from build123d import *

# Parameters (mm, degrees)
SKETCH1_W           = 100
SKETCH1_H           = 320
SKETCH1_R           = 1.6
SKETCH1_W_2         = 50
SKETCH1_H_2         = 280
BOSS_EXTRUDE1_DEPTH = 5
SKETCH2_W           = 50
SKETCH2_H           = 320
BOSS_EXTRUDE2_DEPTH = 5
SKETCH3_W           = 25
SKETCH3_H           = 320
BOSS_EXTRUDE3_DEPTH = 5
CUT_EXTRUDE1_REACH  = 7
SKETCH4_R           = 1.6


with BuildPart() as part:
    # Sketch1 → Boss-Extrude1 (new body)
    with BuildSketch(Plane.XY):
        Rectangle(SKETCH1_W, SKETCH1_H)
        with Locations((-22.5, 145)):
            Circle(SKETCH1_R, mode=Mode.SUBTRACT)
        with Locations((-22.5, 155)):
            Circle(SKETCH1_R, mode=Mode.SUBTRACT)
        with Locations((22.5, 145)):
            Circle(SKETCH1_R, mode=Mode.SUBTRACT)
        with Locations((22.5, -145)):
            Circle(SKETCH1_R, mode=Mode.SUBTRACT)
        with Locations((-22.5, -145)):
            Circle(SKETCH1_R, mode=Mode.SUBTRACT)
        with Locations((22.5, 155)):
            Circle(SKETCH1_R, mode=Mode.SUBTRACT)
        with Locations((22.5, -155)):
            Circle(SKETCH1_R, mode=Mode.SUBTRACT)
        with Locations((-22.5, -155)):
            Circle(SKETCH1_R, mode=Mode.SUBTRACT)
        Rectangle(SKETCH1_W_2, SKETCH1_H_2, mode=Mode.SUBTRACT)
    extrude(amount=BOSS_EXTRUDE1_DEPTH)

    # Sketch2 → Boss-Extrude2 (add)
    with BuildSketch(Plane.XY):
        with Locations((75, 0)):
            Rectangle(SKETCH2_W, SKETCH2_H)
    extrude(amount=BOSS_EXTRUDE2_DEPTH)

    # Sketch3 → Boss-Extrude3 (add)
    with BuildSketch(Plane.XY):
        with Locations((-62.5, 0)):
            Rectangle(SKETCH3_W, SKETCH3_H)
    extrude(amount=BOSS_EXTRUDE3_DEPTH)

    # Sketch4 → Cut-Extrude1 (cut, up to next)
    with BuildSketch(Plane.XY.offset(5), mode=Mode.PRIVATE) as cut_extrude1_sk1:
        with Locations((-60, 75)):
            Circle(SKETCH4_R)
    cut_extrude1_tool1 = extrude(cut_extrude1_sk1.sketch, amount=-CUT_EXTRUDE1_REACH, mode=Mode.PRIVATE) & part.part
    add(cut_extrude1_tool1.solids().sort_by_distance((-60, 75, 5))[0], mode=Mode.SUBTRACT)
    # Sketch4 → Cut-Extrude1 (cut, up to next)
    with BuildSketch(Plane.XY.offset(5), mode=Mode.PRIVATE) as cut_extrude1_sk2:
        with Locations((-60, 60)):
            Circle(SKETCH4_R)
    cut_extrude1_tool2 = extrude(cut_extrude1_sk2.sketch, amount=-CUT_EXTRUDE1_REACH, mode=Mode.PRIVATE) & part.part
    add(cut_extrude1_tool2.solids().sort_by_distance((-60, 60, 5))[0], mode=Mode.SUBTRACT)
    # Sketch4 → Cut-Extrude1 (cut, up to next)
    with BuildSketch(Plane.XY.offset(5), mode=Mode.PRIVATE) as cut_extrude1_sk3:
        with Locations((-60, -60)):
            Circle(SKETCH4_R)
    cut_extrude1_tool3 = extrude(cut_extrude1_sk3.sketch, amount=-CUT_EXTRUDE1_REACH, mode=Mode.PRIVATE) & part.part
    add(cut_extrude1_tool3.solids().sort_by_distance((-60, -60, 5))[0], mode=Mode.SUBTRACT)
    # Sketch4 → Cut-Extrude1 (cut, up to next)
    with BuildSketch(Plane.XY.offset(5), mode=Mode.PRIVATE) as cut_extrude1_sk4:
        with Locations((-60, -75)):
            Circle(SKETCH4_R)
    cut_extrude1_tool4 = extrude(cut_extrude1_sk4.sketch, amount=-CUT_EXTRUDE1_REACH, mode=Mode.PRIVATE) & part.part
    add(cut_extrude1_tool4.solids().sort_by_distance((-60, -75, 5))[0], mode=Mode.SUBTRACT)
    # Sketch4 → Cut-Extrude1 (cut, up to next)
    with BuildSketch(Plane.XY.offset(5), mode=Mode.PRIVATE) as cut_extrude1_sk5:
        with Locations((85, -75)):
            Circle(SKETCH4_R)
    cut_extrude1_tool5 = extrude(cut_extrude1_sk5.sketch, amount=-CUT_EXTRUDE1_REACH, mode=Mode.PRIVATE) & part.part
    add(cut_extrude1_tool5.solids().sort_by_distance((85, -75, 5))[0], mode=Mode.SUBTRACT)
    # Sketch4 → Cut-Extrude1 (cut, up to next)
    with BuildSketch(Plane.XY.offset(5), mode=Mode.PRIVATE) as cut_extrude1_sk6:
        with Locations((85, -60)):
            Circle(SKETCH4_R)
    cut_extrude1_tool6 = extrude(cut_extrude1_sk6.sketch, amount=-CUT_EXTRUDE1_REACH, mode=Mode.PRIVATE) & part.part
    add(cut_extrude1_tool6.solids().sort_by_distance((85, -60, 5))[0], mode=Mode.SUBTRACT)
    # Sketch4 → Cut-Extrude1 (cut, up to next)
    with BuildSketch(Plane.XY.offset(5), mode=Mode.PRIVATE) as cut_extrude1_sk7:
        with Locations((85, 60)):
            Circle(SKETCH4_R)
    cut_extrude1_tool7 = extrude(cut_extrude1_sk7.sketch, amount=-CUT_EXTRUDE1_REACH, mode=Mode.PRIVATE) & part.part
    add(cut_extrude1_tool7.solids().sort_by_distance((85, 60, 5))[0], mode=Mode.SUBTRACT)
    # Sketch4 → Cut-Extrude1 (cut, up to next)
    with BuildSketch(Plane.XY.offset(5), mode=Mode.PRIVATE) as cut_extrude1_sk8:
        with Locations((85, 75)):
            Circle(SKETCH4_R)
    cut_extrude1_tool8 = extrude(cut_extrude1_sk8.sketch, amount=-CUT_EXTRUDE1_REACH, mode=Mode.PRIVATE) & part.part
    add(cut_extrude1_tool8.solids().sort_by_distance((85, 75, 5))[0], mode=Mode.SUBTRACT)


solid = part.part
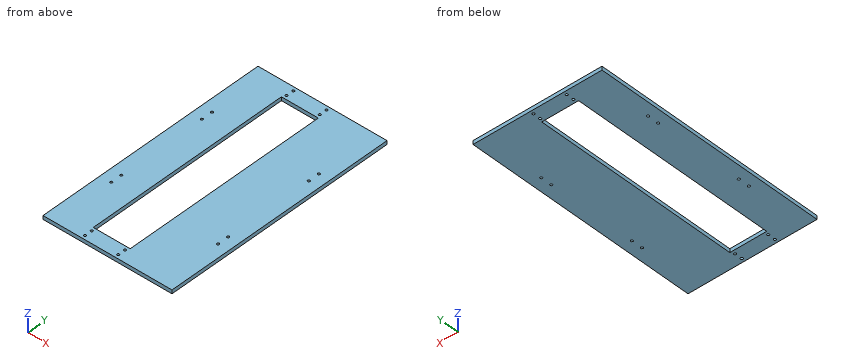
Geometry: final body of the model. Coordinates: model frame, mm. Give positions to 0.01 mm unless a question says otherwise; leave off trailing zeros. Loops run counter-clockwise (first coordinate to the right, second up) from the corner with the lowest first, then second, coordinate; pieces in that order, holes last. Notation, with made-up numbers: M 43.25,37 L 87.25,37 A7 cw 87.25,45 Z; hole C -9.75,46 d3. An arc over 180 degrees is marked long. Put each result on its own line as item: value.
1) Cut plane A-A, the plane y = -31. Return the cut outline in (x, z).
Computed values:
outline: M -75,0 L -25,0 L -25,5 L -75,5 Z; M 25,0 L 100,0 L 100,5 L 25,5 Z
2) Cut plane B-B, the plane x = -0.5. Return the cut outline in (y, z).
Computed values:
outline: M -160,0 L -140,0 L -140,5 L -160,5 Z; M 140,0 L 160,0 L 160,5 L 140,5 Z
3) Cut plane C-C, the plane z = 0.75. Give the number of separate pieces and of enclosed holes in the cut face, plus the area to 3 significant figures.
Computed values:
separate pieces: 1
enclosed holes: 17
area: 41,900 mm^2
4) Material intervals for L1, parallel to X at y = 75, z = 1.7; L2, parallel to Y at x = 85, z = 2.9; L3, parallel to X at y = -145, z = 3.45, sorted ascending. Write a range as from..to.
Computed values:
L1: x = -75..-61.6, -58.4..-25, 25..83.4, 86.6..100
L2: y = -160..-76.6, -73.4..-61.6, -58.4..58.4, 61.6..73.4, 76.6..160
L3: x = -75..-24.1, -20.9..20.9, 24.1..100
5) First-contact query: P1, Ø1.9, axis at x = -22.5, y = 145, coming from the -Z side. Flat tip, straight axial feed; report the tip coordinate or a pass-through.
Computed values:
P1: passes through
